The listing builds one solid part. Answer for the finished solid, in the listing's coordinates (mm). Face numbers are marked on the shaded views. A direction names the side the tool comes from. Give positions to 0.01 mm unless a question says otherwise; leave off trailing zeros. Loops run counter-clockwise (first coordinate to the right, second up) from the corner with the lowest first, then second, coordinate; pieces in that order, holes last. Notation, with made-up numbers: (30, -14) - (49, -14) arc R20 ccw to (49, -5) - close; hole circle Ø8 at (69, 75.5). An arc over 180 degrees is marked (long way). Answer as CSV lines item,"result". Start each with the question number.
1) Find the intervals of material crossed by line 1 along X through (y, z) = (1.8, -0.85); line 2 along Z through (x, y) = (-8.5, 0.1); line 3 along X through (y, z) = (2.3, 1.35), in increasing order.
2) For the marked faces 1 and 2, determine the directions among +Z, -Z, +X, -X, +Y, -Y from which every point of the face is accessible in a straight line to the end or side of a thin tool.
3) A cutting plane is placed at A-A (z = 0). Determine the outline of the cut face in (x, y) (3 decimals), and give its area (3 significant figures).
4) A cutting plane is placed at B-B (x = -7). Determine the outline of the cut face in (y, z), and give its area (3 significant figures).
5) A flat-ended cylindrical pin translates along its axis: pin 1 (1 mm diameter, centred on x = -7, y = 1.5, fed in from -Z). Find the tip coordinate at first contact, or state that the pin passes through.
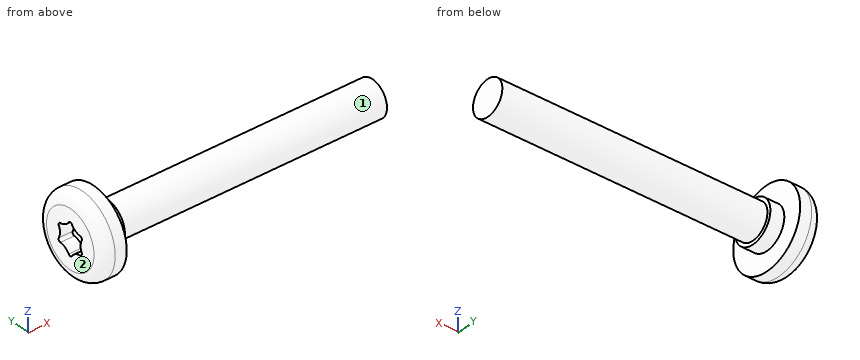
```python
from build123d import *

# Parameters (mm, degrees)
EXTRUDE1_DEPTH    = 1
FILLET1_R         = 0.825
FILLET2_R         = 0.162857143
SKETCH3_OUTSIDE_W = 12.32
SKETCH3_OUTSIDE_H = 12.32
SKETCH3_OUTSIDE_R = 1.25
SIS_KIERRE_DEPTH  = 19


with BuildPart() as part:
    # Sketch1 → Revolve1 (revolve)
    with BuildSketch(Plane.XY, mode=Mode.PRIVATE) as revolve1_sk:
        Polygon((-20, 2.85), (-21.65, 2.85), (-21.65, 0), (0, 0), (0, 1.5), (-20, 1.5), align=None)
    revolve(revolve1_sk.sketch.rotate(Axis((22.773389601, 0, 0), (-1, 0, 0)), 90), axis=Axis((22.773389601, 0, 0), (-1, 0, 0)))

    # Sketch2 → Extrude1 (cut)
    with BuildSketch(Plane.ZY.offset(21.65)):
        with BuildLine():
            ThreePointArc((-1.4, 0), (-0.761857658, 0.439858724), (-0.7, 1.212435565))
            ThreePointArc((-0.7, 1.212435565), (0, 0.879717448), (0.7, 1.212435565))
            ThreePointArc((0.7, 1.212435565), (0.761857658, 0.439858724), (1.4, 0))
            ThreePointArc((1.4, 0), (0.761857658, -0.439858724), (0.7, -1.212435565))
            ThreePointArc((0.7, -1.212435565), (0, -0.879717448), (-0.7, -1.212435565))
            ThreePointArc((-0.7, -1.212435565), (-0.761857658, -0.439858724), (-1.4, 0))
        make_face()
    extrude(amount=-EXTRUDE1_DEPTH, mode=Mode.SUBTRACT)

    # Fillet1
    fillet1_edges = [part.edges().sort_by_distance(p)[0] for p in [
        (-21.65, 0, 2.85),
    ]]
    fillet(fillet1_edges, radius=FILLET1_R)

    # Fillet2
    fillet2_edges = [part.edges().sort_by_distance(p)[0] for p in [
        (-21.15, 0, -1.4),
        (-21.15, 1.212435565, -0.7),
        (-21.15, 1.212435565, 0.7),
        (-21.15, 0, 1.4),
        (-21.15, -1.212435565, 0.7),
        (-21.15, -1.212435565, -0.7),
    ]]
    fillet(fillet2_edges, radius=FILLET2_R)

    # Sketch3 outside → Sisäkierre (cut)
    with BuildSketch(Plane(origin=(0, 0, 0), x_dir=(0, 0, -1), z_dir=(1, 0, 0))):
        Rectangle(SKETCH3_OUTSIDE_W, SKETCH3_OUTSIDE_H)
        Circle(SKETCH3_OUTSIDE_R, mode=Mode.SUBTRACT)
    extrude(amount=-SIS_KIERRE_DEPTH, mode=Mode.SUBTRACT)


solid = part.part
```
Ans:
1,line 1,"-21.65 to -20"
1,line 2,"-1.25 to 1.25"
1,line 3,"-21.34 to -20"
2,face 1,"+X"
2,face 2,"+Z, -Z, -X, +Y, -Y"
3,outline,"(-21.65, -2.025) arc R0.825 ccw to (-20.825, -2.85) - (-20, -2.85) - (-20, -1.5) - (-19, -1.5) - (-19, -1.25) - (0, -1.25) - (0, 1.25) - (-19, 1.25) - (-19, 1.5) - (-20, 1.5) - (-20, 2.85) - (-20.825, 2.85) arc R0.825 ccw to (-21.65, 2.025) - (-21.65, 0.88) - (-20.65, 0.88) - (-20.65, -0.88) - (-21.65, -0.88) - close"
3,area,"57.9 mm2"
4,outline,"circle Ø2.5 at (0, 0)"
4,area,"4.91 mm2"
5,pin 1,"z = -0.75"
